Source: three-view drawing plus pictorial views. Frame: mm from the lowest corner of the part. Give positions to 0.01 mm unless a question says otherwise; leave off trailing zeros. Write each loop counter-clockwise with the first axis right and the second up, starting at its lowest first coordinate (ties: lowest second). Pieces come first, ordered by that corner, then holes. Notation, with made-up numbers: M -9.75,-34.75 L 23.25,-34.75 A19 ccw 23.25,-2.75 Z; hole C 89,-9.75 d1. An arc over 180 degrees is marked long. One line per question, with ' | ' between items.
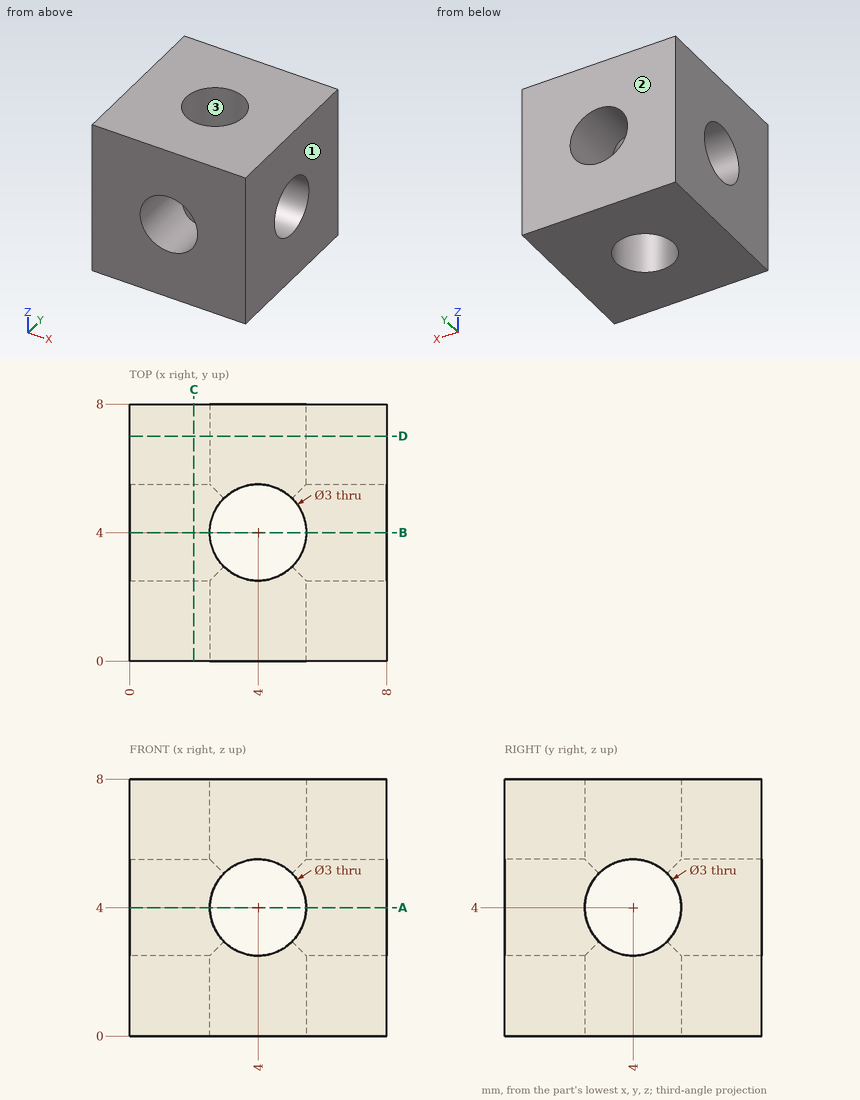
(1) Draft query along X for the marked faces 1, 2 and 3. Return one class per face: released by +X, released by -X, zero draft, split by the parting line, or undercut.
Working result:
face 1: released by +X | face 2: zero draft | face 3: undercut
(2) Cut plane A-A, the plane z = 4. Return loops of the section in (x, y), then the cut area to 3 significant figures.
Working result:
outline: M 0,0 L 2.5,0 L 2.5,2.5 L 0,2.5 Z; M 0,5.5 L 2.5,5.5 L 2.5,8 L 0,8 Z; M 5.5,0 L 8,0 L 8,2.5 L 5.5,2.5 Z; M 5.5,5.5 L 8,5.5 L 8,8 L 5.5,8 Z | area: 25.0 mm^2
(3) Cut plane C-C, the plane x = 2. Return loops of the section in (y, z), then the cut area to 3 significant figures.
Working result:
outline: M 0,0 L 8,0 L 8,8 L 0,8 Z; hole C 4,4 d3 | area: 56.9 mm^2
(4) Material intervals for L1, parallel to Y at x = 4, z = 6.3, sorted ascending. Write a range as [from, to].
Working result:
L1: y = [0, 2.5], [5.5, 8]
